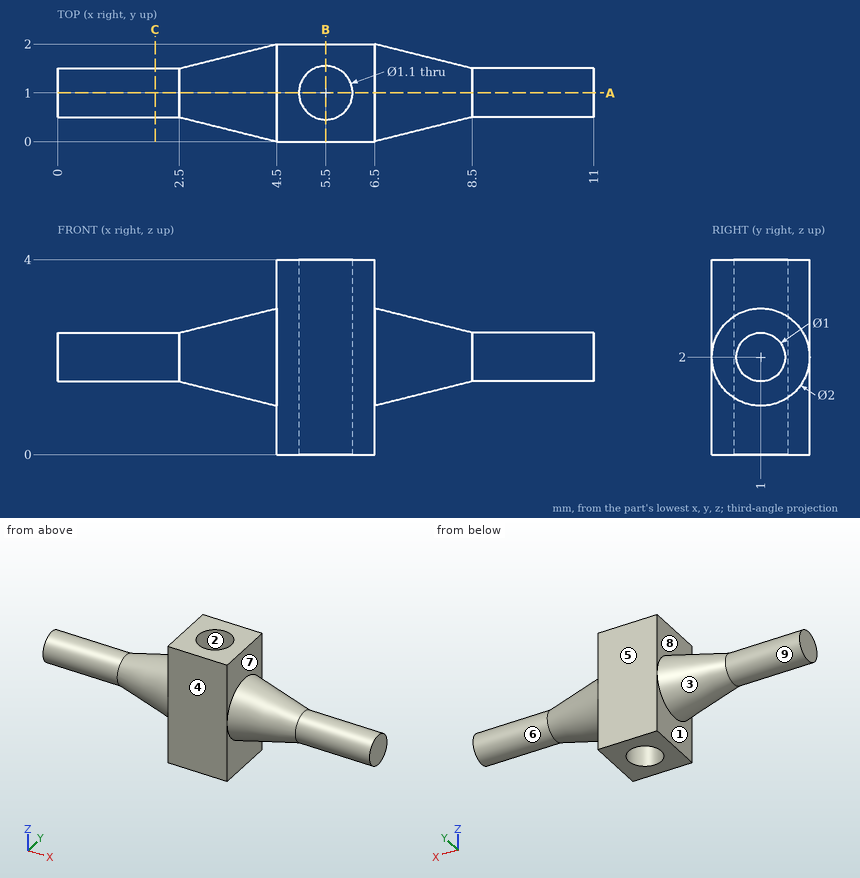
Here's the drawing with two shaded views (mm, measured from the low corner). I have some questions. A direction names the side the tool comes from. Give positions to 0.01 mm unless a question says otherwise; leave off trailing zeros. Loops run counter-clockwise (first coordinate to the right, second up) from the corner with the lowest first, then second, coordinate; pieces in that order, holes last. Notation, with made-up numbers: (18.5, 13) -> (53.5, 13) arc R26 cw to (53.5, 39) -> close; hole circle Ø10 at (4.25, 54.5). An arc over 180 degrees is marked (long way). One line per item, written item: value.
Q1. On a 3-axis mill with a long thin cutter (end or side, diameter ignored), from which of +Z, -Z, +X, -X, +Y, -Y can I reach the whole of each face in a straight line? I mean the marked faces 5, 6, 7, 8 and 9. Say none if no direction works.
Answers follow:
face 5: +Z, -Z, +X, -X, +Y
face 6: +X
face 7: +Z, +X
face 8: +Z, -X
face 9: -X
Q2. I'm going to push a flat-ended pin straight in: pin 1 Ø0.6 at (y, z) = (1, 0.5) entering from +X. Where does the tip first touch, or does it pass through?
Answers follow:
pin 1: x = 6.5
Q3. Suppose I cut it at A-A on y = 1. Please give me the cut outline in (x, z), then the cut area to 3 significant figures.
Answers follow:
outline: (0, 1.5) -> (2.5, 1.5) -> (4.5, 1) -> (4.5, 0) -> (4.95, 0) -> (4.95, 4) -> (4.5, 4) -> (4.5, 3) -> (2.5, 2.5) -> (0, 2.5) -> close; (6.05, 0) -> (6.5, 0) -> (6.5, 1) -> (8.5, 1.5) -> (11, 1.5) -> (11, 2.5) -> (8.5, 2.5) -> (6.5, 3) -> (6.5, 4) -> (6.05, 4) -> close
area: 14.6 mm^2
Q4. If I drill on line 1 along Y through (x, z) = (5.5, 2.2); line 2 along X through (y, z) = (1.9, 3.4); line 3 along X through (y, z) = (1.2, 3.6), over which ranges is the centre line in solid material (lowest first)?
Answers follow:
line 1: 0 to 0.45, 1.55 to 2
line 2: 4.5 to 6.5
line 3: 4.5 to 4.99, 6.01 to 6.5
Q5. Suppose I cut it at C-C on x = 2. Please give me the cut outline in (y, z).
Answers follow:
outline: circle Ø1 at (1, 2)
Q6. Suppose I cut it at B-B on x = 5.5. Please give me the cut outline in (y, z).
Answers follow:
outline: (0, 0) -> (0.45, 0) -> (0.45, 4) -> (0, 4) -> close; (1.55, 0) -> (2, 0) -> (2, 4) -> (1.55, 4) -> close
Q7. We'd pull the mould along Y, two halves only. Please class the marked faces 1, 2, 3 and 4: pulls with the +Y half, pulls with the -Y half, needs draft (parallel to the pull), parting line crosses it, or undercut.
Answers follow:
face 1: needs draft
face 2: undercut
face 3: parting line crosses it
face 4: pulls with the -Y half
